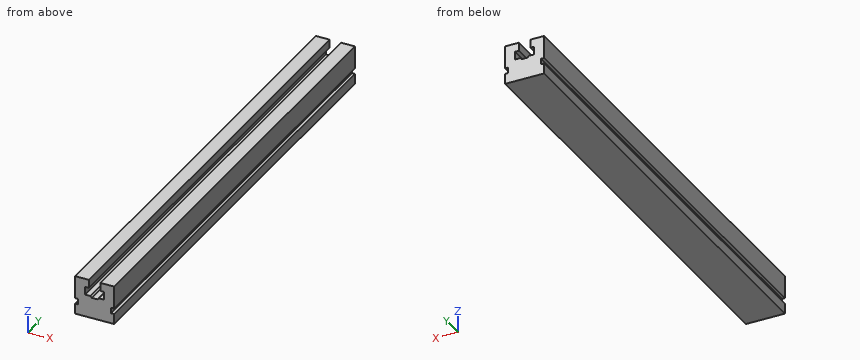
from build123d import *

# Parameters (mm, degrees)
BOSS_EXTRUDE1_DEPTH = 900


with BuildPart() as part:
    # Sketch1 → Boss-Extrude1 (new body)
    with BuildSketch(Plane(origin=(0, 0, 0), x_dir=(1, 0, 0), z_dir=(0, 1, 0))):
        Polygon((37.5, 0), (-37.5, 0), (-37.5, -20), (-32, -20), (-32, -31), (-37.5, -31), (-37.5, -75), (-11, -75), (-11, -58.9), (-18.5, -58.9), (-18.5, -43.4), (-8.4, -43.4), (-5.5, -40.5), (5.5, -40.5), (8.4, -43.4), (18.5, -43.4), (18.5, -58.9), (11, -58.9), (11, -75), (37.5, -75), (37.5, -31), (32, -31), (32, -20), (37.5, -20), align=None)
    extrude(amount=-BOSS_EXTRUDE1_DEPTH)


solid = part.part
Input: part model. Units: mm. Frame: model coordinates. Round coordinates to 2 decimals unless told otherwise and drop trailing zeros. Write each loop counter-clockwise with the first axis right and the second up, starting at its lowest first coordinate (ties: lowest second). Pieces come first, ordered by that corner, then holes.
1) Cut plane A-A (y = -635.5). Return the cut outline in (x, z), then the cut area to 3 significant figures.
2) Ray query, L1, parallel to X at y = -47.5, z = 58.5; L2, parallel to Z at x = -34, y = -222.5; L3, parallel to Z at x = -15, y = -431. Return the intervals inside material, ascending.
3) Contact query for a flat-ended pin moving along its axis: P1, Ø12, axis at x = 2, y = -570.5, coming from the +Z side. Output: stop coordinate, or through.
Geometry says:
1. outline: (-37.5, 0) - (37.5, 0) - (37.5, 20) - (32, 20) - (32, 31) - (37.5, 31) - (37.5, 75) - (11, 75) - (11, 58.9) - (18.5, 58.9) - (18.5, 43.4) - (8.4, 43.4) - (5.5, 40.5) - (-5.5, 40.5) - (-8.4, 43.4) - (-18.5, 43.4) - (-18.5, 58.9) - (-11, 58.9) - (-11, 75) - (-37.5, 75) - (-37.5, 31) - (-32, 31) - (-32, 20) - (-37.5, 20) - close
1. area: 4,540 mm2
2. L1: x = -37.5 to -18.5, 18.5 to 37.5
2. L2: z = 0 to 20, 31 to 75
2. L3: z = 0 to 43.4, 58.9 to 75
3. P1: stops at z = 43
